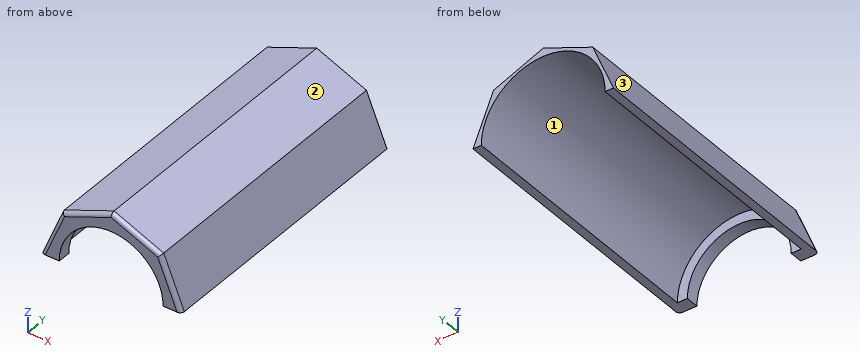
from build123d import *

# Parameters (mm, degrees)
BOSS_EXTRUDE1_DEPTH = 140
SKETCH2_R           = 31
CUT_EXTRUDE1_DEPTH  = 133.5
SKETCH3_R           = 26
CUT_EXTRUDE2_DEPTH  = 133.5
FILLET1_R           = 2
CUT_EXTRUDE3_DEPTH  = 173.5


with BuildPart() as part:
    # Sketch1 → Boss-Extrude1 (new body)
    with BuildSketch(Plane(origin=(0, 0, 0), x_dir=(1, 0, 0), z_dir=(0, 1, 0))):
        Polygon((35.15, 0), (24.854803359, 24.854803359), (0, 35.15), (-24.854803359, 24.854803359), (-35.15, 0), (-24.854803359, -24.854803359), (0, -35.15), (24.854803359, -24.854803359), align=None)
    extrude(amount=BOSS_EXTRUDE1_DEPTH)

    # Sketch2 → Cut-Extrude1 (cut)
    with BuildSketch(Plane(origin=(0, 140, 0), x_dir=(1, 0, 0), z_dir=(0, 1, 0))):
        with Locations(Location((0, 0, 0), (0, 0, 270))):
            Circle(SKETCH2_R)
    extrude(amount=-CUT_EXTRUDE1_DEPTH, mode=Mode.SUBTRACT)

    # Sketch3 → Cut-Extrude2 (cut)
    with BuildSketch(Plane(origin=(0, 0, 0), x_dir=(-1, 0, 0), z_dir=(0, -1, 0))):
        with Locations(Location((0, 0, 0), (0, 0, 90))):
            Circle(SKETCH3_R)
    extrude(amount=-CUT_EXTRUDE2_DEPTH, mode=Mode.SUBTRACT)

    # Fillet1
    fillet1_edges = [part.edges().sort_by_distance(p)[0] for p in [
        (30.002401679, 0, -12.427401679),
        (30.002401679, 0, 12.427401679),
        (12.427401679, 0, 30.002401679),
        (-12.427401679, 0, 30.002401679),
        (-30.002401679, 0, 12.427401679),
        (-30.002401679, 0, -12.427401679),
        (-12.427401679, 0, -30.002401679),
        (12.427401679, 0, -30.002401679),
    ]]
    fillet(fillet1_edges, radius=FILLET1_R)

    # Sketch4 → Cut-Extrude3 (cut)
    with BuildSketch(Plane(origin=(0, 140, 0), x_dir=(1, 0, 0), z_dir=(0, 1, 0))):
        Polygon((-35.15, 0), (35.15, 0), (24.854803359, 24.854803359), (0, 35.15), (-24.854803359, 24.854803359), align=None)
    extrude(amount=-CUT_EXTRUDE3_DEPTH, mode=Mode.SUBTRACT)


solid = part.part
The listing builds one solid part. Answer for the finished solid, in the listing's coordinates (mm). Face numbers are marked on the shaded views. Round coordinates to 2 decimals unless told otherwise and drop trailing zeros. Write each loop counter-clockwise with the first axis right and the second up, starting at its lowest first coordinate (ties: lowest second). Pieces come first, ordered by that corner, then holes. Notation, with made-up numbers: M 73.25,80 L 118.25,80 A12 ccw 118.25,90 Z; hole C 6,9.25 d8. An arc over 180 degrees is marked long. Write each question's results on one line, items separated by ' | '. Start each with the question number.
(1) The part is cut by section A-A, the plane y = 14.5. Write down the section's boundary in (x, z).
(2) Each of these flat-tipped pins is pushed along its axis until it touches: P1, Ø1.5, axis at x = -6, y = 86, coming from the -Z side; P2, Ø1, axis at x = -26.5, y = 84, coming from the +Z side; P3, Ø10, axis at x = -3.5, y = 63.5, coming from the +Z side. Where does it stop, or does it pass through?
(3) Determine the mould class of the marked faces 1, 2 and 3 for opening direction X: +X half, -X half, draft (parallel to the pull), parting line (faces both ways), or undercut.
(4) Find the intervals of material crossed by line 1 (X direction, y = 48, z = 27); line 2 (X direction, y = 120, z = 6); line 3 (Y direction, x = 21, z = 21.5), in increasing order.
Worked answers:
1) outline: M -35.15,0 L -31,0 A31 cw 31,0 L 35.15,0 L 24.85,24.85 L 0,35.15 L -24.85,24.85 Z
2) P1: stops at z = 30.26 | P2: stops at z = 22.09 | P3: stops at z = 35.15
3) face 1: undercut | face 2: +X half | face 3: -X half
4) line 1: x = -19.68 to -15.23, 15.23 to 19.68 | line 2: x = -32.66 to -30.41, 30.41 to 32.66 | line 3: y = 0 to 6.5
